Read the model definition and answer for the solid it produces. Units are mm, in the model's axes. A direction names the side the tool comes from. Coordinates: 2 decimals unless noted, no trailing zeros. Order: outer loops, then holes, each group sorted by start corner. A loop starts at its lowest first (then second) coordinate and runs counter-clockwise, first axis right, second up. Notation, with made-up numbers: (38.5, -11.75) -> (82.5, -11.75) arc R30 ccw to (82.5, 23.25) -> close; hole circle Ø7 at (-25.5, -30). An arc over 180 degrees is marked (long way). Answer in a Markdown table with one row per item.
from build123d import *
from OCP.BRepFilletAPI import BRepFilletAPI_MakeChamfer

# Parameters (mm, degrees)
BOSS_EXTRUDE1_DEPTH      = 6
BOSS_EXTRUDE1_DEPTH_BACK = 6
CUT_EXTRUDE1_DEPTH       = 157
CUT_EXTRUDE4_DEPTH       = 2.5
CUT_EXTRUDE4_DEPTH_BACK  = 2.5
SKETCH8_W                = 125
SKETCH8_H                = 34.7
CUT_EXTRUDE5_DEPTH       = 131.348014108
CUT_EXTRUDE5_DEPTH_BACK  = 131.348014108
SKETCH9_R                = 2.7
CHAMFER2_SIZE            = 5
CHAMFER2_SIZE_2          = 0.262038896
CUT_EXTRUDE8_DEPTH       = 10
CUT_EXTRUDE9_DEPTH       = 131.715773363
SKETCH16_W               = 214.344642296
SKETCH16_H               = 84.645654919
CUT_EXTRUDE10_DEPTH      = 131.348014108
SKETCH17_W               = 2
SKETCH17_H               = 14.7
CUT_EXTRUDE11_DEPTH      = 1.8
SKETCH18_R               = 1.35
CUT_EXTRUDE12_DEPTH      = 3
CHAMFER7_SIZE            = 3.5
SKETCH19_W               = 5
SKETCH19_H               = 7.5
BOSS_EXTRUDE2_DEPTH      = 2


with BuildPart() as part:
    # Sketch1 → Boss-Extrude1 (new, two sides: drawn at the far end of the back side and taken through both)
    with BuildSketch(Plane.XY.offset(-BOSS_EXTRUDE1_DEPTH_BACK)):
        Polygon((-127.819104229, -9.862903226), (22.180895771, -9.862903226), (22.180895771, -2.612903226), (27.180895771, -2.612903226), (27.180895771, 2.887096774), (22.180895771, 2.887096774), (22.180895771, 10.137096774), (31.180895771, 10.137096774), (31.180895771, 23.637096774), (31.180895771, 24.837096774), (-88.819104229, 24.837096774), (-88.819104229, 23.637096774), (-88.819104229, 15.637096774), (-127.819104229, 15.637096774), align=None)
    extrude(amount=BOSS_EXTRUDE1_DEPTH + BOSS_EXTRUDE1_DEPTH_BACK)

    # Sketch2 → Cut-Extrude1 (cut)
    with BuildSketch(Plane.ZY.offset(127.819104229)):
        Polygon((-4.8, 23.137096774), (-4.8, 8.137096774), (4.8, 8.137096774), (4.8, 23.137096774), (1.8, 23.137096774), (1.8, 24.837096774), (-1.8, 24.837096774), (-1.8, 23.137096774), align=None)
    extrude(amount=-CUT_EXTRUDE1_DEPTH, mode=Mode.SUBTRACT)

    # Sketch8 → Cut-Extrude4 (cut, two sides: drawn at the far end of the back side and taken through both)
    with BuildSketch(Plane.XY.offset(-CUT_EXTRUDE4_DEPTH_BACK)):
        with Locations((-45.319104229, 7.487096774)):
            Rectangle(SKETCH8_W, SKETCH8_H)
    extrude(amount=CUT_EXTRUDE4_DEPTH + CUT_EXTRUDE4_DEPTH_BACK, mode=Mode.SUBTRACT)

    # Sketch9 → Cut-Extrude5 (cut, two sides: drawn at the far end of the back side and taken through both)
    with BuildSketch(Plane.XY.offset(-CUT_EXTRUDE5_DEPTH_BACK)):
        with Locations((-77.819104229, -0.862903226)):
            Circle(SKETCH9_R)
        with Locations((2.180895771, -0.862903226)):
            Circle(SKETCH9_R)
    extrude(amount=CUT_EXTRUDE5_DEPTH + CUT_EXTRUDE5_DEPTH_BACK, mode=Mode.SUBTRACT)

    # Chamfer2
    chamfer2_edges_1 = [part.edges().sort_by_distance(p)[0] for p in [
        (27.180895771, -2.612903226, 0),
    ]]
    chamfer2_side_1 = [part.faces().sort_by_distance(p)[0] for p in [
        (27.175654993, -2.612903226, 0),
    ]]
    chamfer2_edges_2 = [part.edges().sort_by_distance(p)[0] for p in [
        (27.180895771, 2.887096774, 0),
    ]]
    chamfer2_side_2 = [part.faces().sort_by_distance(p)[0] for p in [
        (27.180895771, 2.881855996, 0),
    ]]
    chamfer2 = BRepFilletAPI_MakeChamfer(part.part.solid().wrapped)
    for e in chamfer2_edges_1:
        chamfer2.Add(CHAMFER2_SIZE - 0.0001, CHAMFER2_SIZE_2 - 0.0001, e.wrapped, chamfer2_side_1[0].wrapped)
    for e in chamfer2_edges_2:
        chamfer2.Add(CHAMFER2_SIZE_2 - 0.0001, CHAMFER2_SIZE - 0.0001, e.wrapped, chamfer2_side_2[0].wrapped)
    add(Compound.cast(chamfer2.Shape()), mode=Mode.REPLACE)  # a hair under: the kernel refuses the full size

    # Sketch14 → Cut-Extrude8 (cut)
    with BuildSketch(Plane(origin=(0, 8.137096774, 0), x_dir=(1, 0, 0), z_dir=(0, 1, 0))):
        with BuildLine():
            Line((-120.319104229, 4.5), (-115.319104229, 4.5))
            ThreePointArc((-115.319104229, 4.5), (-110.819104229, 0), (-115.319104229, -4.5))
            Line((-115.319104229, -4.5), (-120.319104229, -4.5))
            ThreePointArc((-120.319104229, -4.5), (-124.819104229, 0), (-120.319104229, 4.5))
        make_face()
    extrude(amount=-CUT_EXTRUDE8_DEPTH, mode=Mode.SUBTRACT)

    # Sketch15 → Cut-Extrude9 (cut, through all)
    with BuildSketch(Plane(origin=(0, -1.862903226, 0), x_dir=(1, 0, 0), z_dir=(0, 1, 0))):
        with BuildLine():
            Line((-120.319104229, -2.6), (-115.319104229, -2.6))
            ThreePointArc((-115.319104229, -2.6), (-112.719104229, 0), (-115.319104229, 2.6))
            Line((-115.319104229, 2.6), (-120.319104229, 2.6))
            ThreePointArc((-120.319104229, 2.6), (-122.919104229, 0), (-120.319104229, -2.6))
        make_face()
    extrude(amount=-CUT_EXTRUDE9_DEPTH, mode=Mode.SUBTRACT)

    # Sketch16 → Cut-Extrude10 (cut, through all)
    with BuildSketch(Plane.XY):
        with Locations((-30.272765953, 16.776086779)):
            Rectangle(SKETCH16_W, SKETCH16_H)
    extrude(amount=-CUT_EXTRUDE10_DEPTH, mode=Mode.SUBTRACT)

    # Sketch17 → Cut-Extrude11 (cut)
    with BuildSketch(Plane(origin=(0, 0, 0), x_dir=(-1, 0, 0), z_dir=(0, 0, -1))):
        with Locations((-30.180895771, 17.487096774)):
            Rectangle(SKETCH17_W, SKETCH17_H)
    extrude(amount=-CUT_EXTRUDE11_DEPTH, mode=Mode.SUBTRACT)

    # Sketch18 → Cut-Extrude12 (cut)
    with BuildSketch(Plane(origin=(0, 0, 0), x_dir=(-1, 0, 0), z_dir=(0, 0, -1))):
        with Locations((110.319104229, -5.862903226)):
            Circle(SKETCH18_R)
        with Locations((125.319104229, -5.862903226)):
            Circle(SKETCH18_R)
        with Locations((-22.180895771, 0.137096774)):
            Circle(SKETCH18_R)
    extrude(amount=-CUT_EXTRUDE12_DEPTH, mode=Mode.SUBTRACT)

    # Chamfer7
    chamfer7_edges = [part.edges().sort_by_distance(p)[0] for p in [
        (-80.519104229, -0.862903226, 6),
        (-0.519104229, -0.862903226, 6),
    ]]
    chamfer(chamfer7_edges, length=CHAMFER7_SIZE - 0.0001)  # a hair under: the kernel refuses the full size

    # Sketch19 → Boss-Extrude2 (add)
    with BuildSketch(Plane(origin=(0, 0, 4.8), x_dir=(-1, 0, 0), z_dir=(0, 0, -1))):
        with Locations((93.819104229, 11.887096774)):
            Rectangle(SKETCH19_W, SKETCH19_H)
    extrude(amount=BOSS_EXTRUDE2_DEPTH)


solid = part.part
Q1. The part is cut by section B-B (x = -7). Write down the section's boundary in (y, z).
Outcome:
| item | result |
|---|---|
| outline | (-9.86, 2.5) -> (8.14, 2.5) -> (8.14, 4.8) -> (23.14, 4.8) -> (23.14, 2.5) -> (24.84, 2.5) -> (24.84, 6) -> (-9.86, 6) -> close |
Q2. For a pull along Y with two mould halves and no side action, classify faces 4 (the face through (22, 0, 3)), 5 (the face through (21, -1, 0)), 6 (the face through (-118, -1.863, 3)) as pulls with the +Y half, pulls with the -Y half, needs draft (parallel to the pull), parting line crosses it, or undercut.
Outcome:
| item | result |
|---|---|
| face 4 | undercut |
| face 5 | needs draft |
| face 6 | pulls with the +Y half |
Q3. Given pin 1 (1 mm diameter, centred on y = 8.5, z = 3.5, fed in from +X); pin 2 (1.4 mm diameter, centred on x = -46.5, y = 23.5, fed in from -Z); pin 3 (0.8 mm diameter, centred on x = -125.5, y = -5.5, fed in from -Z), each flat-ended and moving along its own axis, determine where each tip first touches the part or whether it passes through.
Outcome:
| item | result |
|---|---|
| pin 1 | x = 22.18 |
| pin 2 | z = 2.5 |
| pin 3 | z = 3 |
Q4. The part is cut by section C-C (y = 19.5). Write down the section's boundary in (x, z).
Outcome:
| item | result |
|---|---|
| outline | (-88.82, 4.8) -> (29.18, 4.8) -> (29.18, 1.8) -> (31.18, 1.8) -> (31.18, 6) -> (-88.82, 6) -> close |
Q5. Consider line 1 (X direction, y = 2.5, z = 1); line 2 (Y direction, x = -45, z = 4.75); line 3 (X direction, y = -1.5, z = 1.5). Determine where each line is inside the solid, lowest interval first.
Outcome:
| item | result |
|---|---|
| line 1 | -127.82 to -124.71, -110.93 to -107.82, 17.18 to 27.18 |
| line 2 | -9.86 to 8.14, 23.14 to 24.84 |
| line 3 | -127.82 to -124.56, -111.08 to -107.82, 17.18 to 27.18 |
Q6. For faces 1 (the face through (27.181, 0, 3)), 2 (the face through (-126.566, -6.38, 1.479)), 3 (the face through (-118, -6, 2.6)), determine the directions among +Z, -Z, +X, -X, +Y, -Y from which every point of the face is accessible in a straight line to the end or side of a thin tool.
Outcome:
| item | result |
|---|---|
| face 1 | +Z, -Z, +X, -Y |
| face 2 | -Z |
| face 3 | -Z, +Y, -Y |
Q7. The part is cut by section A-A (y = 12). Write down the section's boundary in (x, z).
Outcome:
| item | result |
|---|---|
| outline | (-127.82, 4.8) -> (-96.32, 4.8) -> (-96.32, 2.8) -> (-91.32, 2.8) -> (-91.32, 4.8) -> (29.18, 4.8) -> (29.18, 1.8) -> (31.18, 1.8) -> (31.18, 6) -> (-127.82, 6) -> close |
